Solid Edge part; units mm, degrees
sketch "Sketch1" plane through (0, 0, 0) normal (0, 0, 1) x (1, 0, 0)
  line L0 (100, -25) -> (100, 25)
  line L1 (100, 25) -> (-40, 25)
  line L2 (-40, 25) -> (-40, -25)
  line L3 (-40, -25) -> (100, -25)
extrude "Extrusionsausprägung_20" add sketch "Sketch1" along normal blind 40
sketch "Sketch2" plane through (30, 0, 40) normal (0, 0, 1) x (1, 0, 0)
  line L0 (-70, -15.25) -> (30, -15.25)
  line L1 (30, -15.25) -> (30, 15.25)
  line L2 (30, 15.25) -> (-70, 15.25)
  line L3 (-70, 15.25) -> (-70, -15.25)
extrude "Extrusionsausschnitt_24" cut sketch "Sketch2" against normal blind 30
sketch "Sketch3" plane through (30, 0, 40) normal (0, 0, 1) x (1, 0, 0)
  circle A0 centre (50, 0) radius 6.5
extrude "Extrusionsausschnitt_25" cut sketch "Sketch3" against normal blind 78
sketch "Sketch4" plane through (0, 0, 15) normal (0, 0, 1) x (1, 0, 0)
  circle A0 centre (80, 0) radius 12.25
extrude "Extrusionsausschnitt_26" cut sketch "Sketch4" along normal blind 2.8
sketch "Sketch5" plane through (0, 0, 15) normal (0, 0, 1) x (1, 0, 0)
  line L0 (70.45, -5.5137) -> (80, -11.0274)
  line L1 (80, -11.0274) -> (89.55, -5.5137)
  line L2 (89.55, 5.5137) -> (89.55, -5.5137)
  line L3 (80, 11.0274) -> (89.55, 5.5137)
  line L4 (70.45, 5.5137) -> (80, 11.0274)
  line L5 (70.45, 5.5137) -> (70.45, -5.5137)
extrude "Extrusionsausschnitt_28" cut sketch "Sketch5" against normal blind 10.2
fillet "Verrundung_15" radius 5 6 edges at (100, -25, 20) (100, 25, 20) (-40, -25, 20) (-40, -15.25, 25) (-40, 15.25, 25) (-40, 25, 20)
fillet "Verrundung_16" radius 2 2 edges at (60, 15.25, 25) (60, -15.25, 25)
sketch "Sketch6" plane through (30, 0, 0) normal (0, 0, -1) x (1, 0, 0)
  circle A0 centre (-58, 0) radius 3.15
  circle A1 centre (-38, 0) radius 3.15
  circle A2 centre (-13, 0) radius 3.15
  circle A3 centre (7, 0) radius 3.15
extrude "Extrusionsausschnitt_29" cut sketch "Sketch6" against normal blind 70
chamfer "Fase_9" distance 0.5 angle 45 15 edges at (73.5, 0, 40) (30, 25, 40) (-38.4911, 23.5795, 40) (-38.4911, 16.6705, 40) (11.5, 15.25, 40) (59.4142, 14.6642, 40) (60, 0, 40) (59.4142, -14.6642, 40) (11.5, -15.25, 40) (-38.4911, -16.6705, 40) (-38.4911, -23.5795, 40) (30, -25, 40) (98.5355, -23.5355, 40) (100, 0, 40) (98.5355, 23.5355, 40)
chamfer "Fase_10" distance 0.5 angle 45 13 edges at (-31.15, 0, 0) (-11.15, 0, 0) (13.85, 0, 0) (33.85, 0, 0) (73.5, 0, 0) (-40, 0, 0) (-38.5355, 23.5355, 0) (30, 25, 0) (98.5355, 23.5355, 0) (100, 0, 0) (98.5355, -23.5355, 0) (30, -25, 0) (-38.5355, -23.5355, 0)
Model file for the job. Use its own axes, mm. A direction names the side the tool comes from. Coordinates: 2 decimals unless noted, no trailing zeros. Write each loop counter-clockwise with the first axis right and the second up, starting at its lowest first coordinate (ties: lowest second). Pieces come first, ordered by that corner, then holes. Notation, with made-up numbers: (39.25, 3.5) - (45.25, 3.5) arc R28 cw to (45.25, 29.5) - close; hole circle Ø4 at (29.25, 20.25). An arc over 180 degrees is marked (long way). One line per item, written item: value. Start each with the question number.
1. Flat gauge pins, fed straight in: pin 1 (5 mm diameter, centred on x = -8, y = 0, fed in from +Z); pin 2 (13 mm diameter, centred on y = 6, z = 26.5, fed in from -X); pin 3 (3 mm diameter, centred on y = 16.5, z = 33, fed in from -X). Where does each tip first touch, or does it go through?
2. Slice it at B-B (x = -8). Write the cut outline in (y, z), plus the area to 3 significant figures.
3. Probe line 1 (X direction, y = 0, z = 7); line 2 (Y direction, x = 17, z = 6.25); line 3 (Y direction, x = 35, z = 27). List the from-to ranges inside material, lowest first. Write a range as from..to.
4. Slice it at A-A (z = 24). Write the cut outline in (x, y) (3 decimals), plus the area to 3 significant figures.
5. Mould opens along Z. For faces 1 (the flat face through (75.158, 8.232, 9.971)), 2 (the conical face through (-38.205, -23.358, 39.858)), 3 (the conical face through (98.319, 23.246, 0.142)) say: released by +Z, released by -Z, zero draft, split by the parting line, or undercut.
6. Tool access for faces 4 (the cylindrical face through (-11.147, -0.138, 5.184)), 5 (the cylindrical face through (-38.45, 16.63, 24.54)), 6 (the flat face through (89.55, 0, 10)): list every direction of +Z, -Z, +X, -X, +Y, -Y with a clear straight run to the whole face (end or side of a thin tool).
7. Slice it at C-C (y = 0). Count the separate pieces of the cut face and the enclosed holes in it, plus the area to 3 significant figures.
Answers below:
1. pin 1: passes through
1. pin 2: stops at x = 60
1. pin 3: stops at x = -39.47
2. outline: (-25, 0.5) - (-24.5, 0) - (-3.65, 0) - (-3.15, 0.5) - (-3.15, 10) - (-15.25, 10) - (-15.25, 39.5) - (-15.75, 40) - (-24.5, 40) - (-25, 39.5) - close; (3.15, 0.5) - (3.65, 0) - (24.5, 0) - (25, 0.5) - (25, 39.5) - (24.5, 40) - (15.75, 40) - (15.25, 39.5) - (15.25, 10) - (3.15, 10) - close
2. area: 1,020 mm^2
3. line 1: x = -40..-31.15, -24.85..-11.15, -4.85..13.85, 20.15..33.85, 40.15..70.45, 89.55..100
3. line 2: y = -25..-3.15, 3.15..25
3. line 3: y = -25..-15.25, 15.25..25
4. outline: (-39.998, -20.125) arc R5 ccw to (-35, -25) - (95, -25) arc R5 ccw to (100, -20) - (100, 20) arc R5 ccw to (95, 25) - (-35, 25) arc R5 ccw to (-39.998, 20.125) arc R5 ccw to (-35, 15.25) - (58, 15.25) arc R2 cw to (60, 13.25) - (60, -13.25) arc R2 cw to (58, -15.25) - (-35, -15.25) arc R5 ccw to start; hole circle Ø13 at (80, 0)
4. area: 3,790 mm^2
5. face 1: undercut
5. face 2: released by +Z
5. face 3: released by -Z
6. face 4: +Z, -Z
6. face 5: +Z, -X
6. face 6: none
7. separate pieces: 6
7. enclosed holes: 0
7. area: 1,730 mm^2
